For this review, take the finished solid that the model builds, in its own axes (mm). A direction names the side the tool comes from. Coordinates: 2 decimals unless noted, no trailing zeros. Write each loop counter-clockwise with the first axis right and the second up, starting at its lowest first coordinate (ties: lowest second). Pieces come first, ordered by that corner, then holes. Notation, with made-up numbers: M 40.5,63 L 69.5,63 A4 cw 69.5,70 Z; hole C 20.25,24.25 d3. An arc over 180 degrees is marked long. One line per question, with ' | ' between items.
from build123d import *

# Parameters (mm, degrees)
BOSS_EXTRUDE1_DEPTH                            = 10
SKETCH3_W                                      = 46
SKETCH3_H                                      = 6
BOSS_EXTRUDE2_DEPTH                            = 10
CSK_FOR_4_OVAL_HEAD_MACHINE_SCREW1_D           = 3.4544
CSK_FOR_4_OVAL_HEAD_MACHINE_SCREW1_DEPTH       = 25
CSK_FOR_4_OVAL_HEAD_MACHINE_SCREW1_CSINK_D     = 8.3228434
CSK_FOR_4_OVAL_HEAD_MACHINE_SCREW1_CSINK_ANGLE = 82
CSK_FOR_4_OVAL_HEAD_MACHINE_SCREW1_TIP         = 1.037806461
SKETCH7_R                                      = 1.125
CUT_EXTRUDE1_DEPTH                             = 52.725839771
SKETCH8_R                                      = 4
CUT_EXTRUDE2_DEPTH                             = 52.725839771
FILLET1_R                                      = 4.25
FILLET2_R                                      = 3
FILLET3_R                                      = 5
SKETCH9_R                                      = 40
CUT_EXTRUDE3_DEPTH                             = 7.5


# Some blends are built 0.0001 mm under size
with BuildPart() as part:
    # Sketch2 → Boss-Extrude1 (new body)
    with BuildSketch(Plane.XY):
        Polygon((-6, 12.01040764), (-29.875261505, 35.885669145), (-35.885669145, 29.875261505), (-12.01040764, 6), (-12.01040764, -6), (-35.885669145, -29.875261505), (-29.875261505, -35.885669145), (-6, -12.01040764), (6, -12.01040764), (29.875261505, -35.885669145), (35.885669145, -29.875261505), (12.01040764, -6), (12.01040764, 6), (35.885669145, 29.875261505), (29.875261505, 35.885669145), (6, 12.01040764), align=None)
    extrude(amount=BOSS_EXTRUDE1_DEPTH)

    # Sketch3 → Boss-Extrude2 (add)
    with BuildSketch(Plane.XY):
        Rectangle(SKETCH3_W, SKETCH3_H)
    extrude(amount=BOSS_EXTRUDE2_DEPTH)

    # CSK for #4 Oval Head Machine Screw1
    with Locations(Plane.XY.offset(10)):
        with Locations((-30.0520382, 30.0520382), (30.0520382, 30.0520382), (30.0520382, -30.0520382), (-30.0520382, -30.0520382)):
            CounterSinkHole(CSK_FOR_4_OVAL_HEAD_MACHINE_SCREW1_D / 2, CSK_FOR_4_OVAL_HEAD_MACHINE_SCREW1_CSINK_D / 2, depth=CSK_FOR_4_OVAL_HEAD_MACHINE_SCREW1_DEPTH, counter_sink_angle=CSK_FOR_4_OVAL_HEAD_MACHINE_SCREW1_CSINK_ANGLE)
            with Locations((0, 0, -(CSK_FOR_4_OVAL_HEAD_MACHINE_SCREW1_DEPTH + CSK_FOR_4_OVAL_HEAD_MACHINE_SCREW1_TIP / 2))):  # 118° drill point
                Cone(0, CSK_FOR_4_OVAL_HEAD_MACHINE_SCREW1_D / 2, CSK_FOR_4_OVAL_HEAD_MACHINE_SCREW1_TIP, mode=Mode.SUBTRACT)

    # Sketch7 → Cut-Extrude1 (cut, through all)
    with BuildSketch(Plane.XY.offset(10)):
        with Locations((20, 0)):
            Circle(SKETCH7_R)
        with Locations((-20, 0)):
            Circle(SKETCH7_R)
    extrude(amount=-CUT_EXTRUDE1_DEPTH, mode=Mode.SUBTRACT)

    # Sketch8 → Cut-Extrude2 (cut, through all)
    with BuildSketch(Plane.XY.offset(10)):
        Circle(SKETCH8_R)
    extrude(amount=-CUT_EXTRUDE2_DEPTH, mode=Mode.SUBTRACT)

    # Fillet1
    # the kernel refuses this fillet: 4.25 mm, written as the material it takes off along each edge
    with BuildSketch(Plane(origin=(35.885669145, -29.875261505, -10.625), x_dir=(-0.7071067811865225, 0.7071067811865727, 0), z_dir=(0, 0, 1)), Plane(origin=(29.875261505, -35.885669145, -10.625), x_dir=(0.7071067811865693, 0.7071067811865258, 0), z_dir=(0, 0, 1)), Plane(origin=(29.875261505, 35.885669145, -10.625), x_dir=(-0.7071067811865508, -0.7071067811865441, 0), z_dir=(0, 0, 1)), Plane(origin=(35.885669145, 29.875261505, -10.625), x_dir=(-0.7071067811889081, 0.7071067811841868, 0), z_dir=(0, 0, 1))) as fillet1_piece_1:
        with BuildLine():
            CenterArc((FILLET1_R, FILLET1_R), FILLET1_R, 180, 90)
            Line((0, FILLET1_R), (0, 0))
            Line((0, 0), (FILLET1_R, 0))
        make_face()
    extrude(amount=31.25, mode=Mode.SUBTRACT)
    with BuildSketch(Plane(origin=(-29.875261505, 35.885669145, -10.625), x_dir=(0.7071067811862382, -0.7071067811868568, 0), z_dir=(0, 0, 1)), Plane(origin=(-35.885669145, 29.875261505, -10.625), x_dir=(0.7071067811865512, 0.7071067811865438, 0), z_dir=(0, 0, 1)), Plane(origin=(-35.885669145, -29.875261505, -10.625), x_dir=(0.7071067811865503, 0.7071067811865446, 0), z_dir=(0, 0, 1)), Plane(origin=(-29.875261505, -35.885669145, -10.625), x_dir=(-0.7071067811865447, 0.7071067811865505, 0), z_dir=(0, 0, 1))) as fillet1_piece_2:
        with BuildLine():
            CenterArc((FILLET1_R, -FILLET1_R), FILLET1_R, 90, 90)
            Line((0, -FILLET1_R), (0, 0))
            Line((0, 0), (FILLET1_R, 0))
        make_face()
    extrude(amount=31.25, mode=Mode.SUBTRACT)

    # Fillet2
    fillet2_edges = [part.edges().sort_by_distance(p)[0] for p in [
        (23, 3, 5),
        (23, -3, 5),
        (-23, 3, 5),
        (-23, -3, 5),
    ]]
    fillet(fillet2_edges, radius=FILLET2_R - 0.0001)  # a hair under: the kernel refuses the full size

    # Fillet3
    # the kernel refuses this fillet: 5 mm, written as the material it adds along each edge
    with BuildSketch(Plane(origin=(-6, 12.01040764, 0), x_dir=(1, 0, 0), z_dir=(0, 0, 1)), Plane(origin=(6, 12.01040764, 0), x_dir=(0.7071067811865509, 0.707106781186544, 0), z_dir=(0, 0, 1)), Plane(origin=(-12.01040764, 6, 0), x_dir=(-0.7071067811865444, 0.7071067811865508, 0), z_dir=(0, 0, 1)), Plane(origin=(12.01040764, 6, 0), x_dir=(0, -1, 0), z_dir=(0, 0, 1))) as fillet3_piece_1:
        with BuildLine():
            CenterArc((FILLET3_R * 0.414213562373, FILLET3_R), FILLET3_R, 225, 45)
            Line((-FILLET3_R * 0.292893218814, FILLET3_R * 0.292893218814), (0, 0))
            Line((0, 0), (FILLET3_R * 0.414213562373, 0))
        make_face()
    extrude(amount=10)
    with BuildSketch(Plane(origin=(-12.01040764, 3, 0), x_dir=(0, 1, 0), z_dir=(0, 0, 1)), Plane(origin=(-12.01040764, -3, 10), x_dir=(0, -1, 0), z_dir=(0, 0, -1))) as fillet3_piece_2:
        with BuildLine():
            CenterArc((FILLET3_R, FILLET3_R), FILLET3_R, 180, 90)
            Line((0, FILLET3_R), (0, 0))
            Line((0, 0), (FILLET3_R, 0))
        make_face()
    extrude(amount=10)
    with BuildSketch(Plane(origin=(-12.01040764, -6, 0), x_dir=(-0.7071067811865506, -0.7071067811865446, 0), z_dir=(0, 0, 1)), Plane(origin=(-6, -12.01040764, 0), x_dir=(1, 0, 0), z_dir=(0, 0, 1)), Plane(origin=(6, -12.01040764, 0), x_dir=(0.7071067811861392, -0.7071067811869558, 0), z_dir=(0, 0, 1)), Plane(origin=(12.01040764, -6, 0), x_dir=(0, 1, 0), z_dir=(0, 0, 1))) as fillet3_piece_3:
        with BuildLine():
            CenterArc((FILLET3_R * 0.414213562373, -FILLET3_R), FILLET3_R, 90, 45)
            Line((-FILLET3_R * 0.292893218813, -FILLET3_R * 0.292893218813), (0, 0))
            Line((0, 0), (FILLET3_R * 0.414213562373, 0))
        make_face()
    extrude(amount=10)
    with BuildSketch(Plane(origin=(12.01040764, -3, 0), x_dir=(1, 0, 0), z_dir=(0, 0, 1)), Plane(origin=(12.01040764, 3, 10), x_dir=(1, 0, 0), z_dir=(0, 0, -1))) as fillet3_piece_4:
        with BuildLine():
            CenterArc((FILLET3_R, -FILLET3_R), FILLET3_R, 90, 90)
            Line((0, -FILLET3_R), (0, 0))
            Line((0, 0), (FILLET3_R, 0))
        make_face()
    extrude(amount=10)

    # Sketch9 → Cut-Extrude3 (cut)
    with BuildSketch(Plane(origin=(0, 0, 0), x_dir=(-1, 0, 0), z_dir=(0, 0, -1))):
        Circle(SKETCH9_R)
    extrude(amount=-CUT_EXTRUDE3_DEPTH, mode=Mode.SUBTRACT)


solid = part.part
1) We need section B-B on z = 5.75. State the section outline as (x, y) points.
Responses:
outline: M -32.88,-26.87 A4.25 ccw -26.87,-32.88 L -25.12,-31.13 A40 cw -31.13,-25.12 Z; M -32.88,26.87 L -31.13,25.12 A40 cw -25.12,31.13 L -26.87,32.88 A4.25 ccw Z; M 25.12,-31.13 L 26.87,-32.88 A4.25 ccw 32.88,-26.87 L 31.13,-25.12 A40 cw Z; M 25.12,31.13 A40 cw 31.13,25.12 L 32.88,26.87 A4.25 ccw 26.87,32.88 Z; hole C -30.05,-30.05 d3.45; hole C -30.05,30.05 d3.45; hole C 30.05,-30.05 d3.45; hole C 30.05,30.05 d3.45
2) Machinability: for faces 1 (the cylindrical face through (-22.14, -2.1, 8.77)), 2 (the cylindrical face through (31.42, 29, 3.55)), 3 (the flat face through (0, 12.01, 9)), 4 (the flat face through (24.57, 18.56, 7.94)), 5 (the flat face through (-2, -4, 7.5)), which of the approach directions +Z, -Z, +X, -X, +Y, -Y give a long, thin tool a straight path to every point of the face, cutting with its end or side? Answer none if there is none.
Responses:
face 1: +Z, -Z, -X | face 2: +Z, -Z | face 3: +Z, -Z, +Y | face 4: +Z, -Z, +X | face 5: -Z
3) We need section C-C on y = 20.5. State the section outline as (x, z) points.
Responses:
outline: M -26.51,7.5 L -14.49,7.5 L -14.49,10 L -26.51,10 Z; M 14.49,7.5 L 26.51,7.5 L 26.51,10 L 14.49,10 Z
4) Insertion check: pin 1 Ø1.2 at (x, z) = (0.5, 8.5) entering from -Y; pin 2 Ø18.5 at (x, y) = (12.5, -15) entering from -Z; pin 3 Ø1.5 at (y, z) = (-15.5, 8.5) entering from -X; pin 4 Ø3.5 at (x, y) = (20, 0) entering from +Z. Each pin has a flat end and moves straight along its axis. Give the tip position at first contact, or say it passes through.
Responses:
pin 1: y = -12.01 | pin 2: z = 7.5 | pin 3: x = -22.26 | pin 4: z = 10
5) The part is to be moulded in two halves that separate along X. For faces 6 (the flat face through (-19, 3, 9)), 7 (the cylindrical face through (12.898, 6.772, 8.732)), 8 (the flat face through (18.56, -24.57, 7.94)), say which applies: +X half, -X half, draft (parallel to the pull), parting line (faces both ways), or undercut.
Responses:
face 6: draft | face 7: +X half | face 8: undercut
6) We need section A-A on x = 0. State the section outline as (y, z) points.
Responses:
outline: M -12.01,7.5 L -4,7.5 L -4,10 L -12.01,10 Z; M 4,7.5 L 12.01,7.5 L 12.01,10 L 4,10 Z
7) To check wall thickness, follow line 1 along Y through (x, z) = (-20, 8.35) (3 decimals); line 2 along Y through (x, z) = (19.5, 9.25); line 3 along X through (y, z) = (0.5, 9.25). State the ranges of each line that lie inside material, in increasing order. Write a range as [from, to].
Responses:
line 1: [-26.01, -13.99], [-3, -1.125], [1.125, 3], [13.99, 26.01] | line 2: [-25.51, -13.49], [-3, -1.01], [1.01, 3], [13.49, 25.51] | line 3: [-22.96, -21.01], [-18.99, -3.97], [3.97, 18.99], [21.01, 22.96]
